Source: three-view drawing plus pictorial views. Frame: mm from the lowest corner of the part. Give positions to 0.01 mm unless a question says otherwise; leave off trailing zeros. Loops run counter-clockwise (first coordinate to the right, second up) from the corner with the lowest first, then second, coordinate; pieces in that order, holes last.
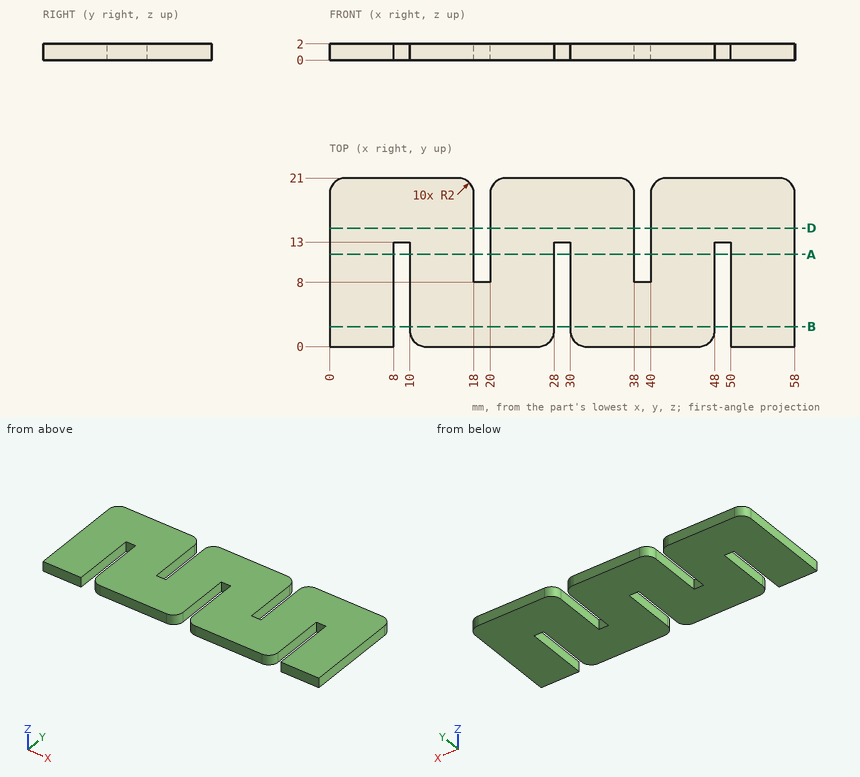
(1) Cut plane A-A (y = 11.5). Return the cut outline in (x, z).
Values follow:
outline: (0, 0) - (8, 0) - (8, 2) - (0, 2) - close; (10, 0) - (18, 0) - (18, 2) - (10, 2) - close; (20, 0) - (28, 0) - (28, 2) - (20, 2) - close; (30, 0) - (38, 0) - (38, 2) - (30, 2) - close; (40, 0) - (48, 0) - (48, 2) - (40, 2) - close; (50, 0) - (58, 0) - (58, 2) - (50, 2) - close
(2) Pin query (flat end, axial travel): pin 1 Ø1 at (x, z) = (21.5, 1.5) entering from +Y; pin 2 Ø1 at (x, z) = (29, 1) entering from -Y. Return the tip coordinate at first contact, or that it passes through.
Values follow:
pin 1: stops at y = 21
pin 2: stops at y = 13
(3) Cut plane B-B (y = 2.5). Return the cut outline in (x, z), and give its area (3 significant figures).
Values follow:
outline: (0, 0) - (8, 0) - (8, 2) - (0, 2) - close; (10, 0) - (28, 0) - (28, 2) - (10, 2) - close; (30, 0) - (48, 0) - (48, 2) - (30, 2) - close; (50, 0) - (58, 0) - (58, 2) - (50, 2) - close
area: 104 mm2
(4) Cut plane D-D (y = 14.75). Return the cut outline in (x, z).
Values follow:
outline: (0, 0) - (18, 0) - (18, 2) - (0, 2) - close; (20, 0) - (38, 0) - (38, 2) - (20, 2) - close; (40, 0) - (58, 0) - (58, 2) - (40, 2) - close
(5) Ray query, probe 1 along X at (y, z) = (9.75, 0.6); probe 2 along X at (y, z) = (6.5, 1.45); probe 3 along X at (y, z) = (1.5, 1.2). Return the intervals inside material, ascending.
Values follow:
probe 1: x = 0 to 8, 10 to 18, 20 to 28, 30 to 38, 40 to 48, 50 to 58
probe 2: x = 0 to 8, 10 to 28, 30 to 48, 50 to 58
probe 3: x = 0 to 8, 10.06 to 27.94, 30.06 to 47.94, 50 to 58
